```python
from build123d import *

# Parameters (mm, degrees)
SKETCH1_W           = 127
SKETCH1_H           = 38.1
BOSS_EXTRUDE1_DEPTH = 6.35
CUT_EXTRUDE1_DEPTH  = 6.35
FILLET1_R           = 30.48
CHAMFER1_SIZE       = 10.16
CHAMFER1_SIZE2      = 3.69793758


with BuildPart() as part:
    # Sketch1 → Boss-Extrude1 (new body)
    with BuildSketch(Plane.XY):
        with Locations((63.5, 19.05)):
            Rectangle(SKETCH1_W, SKETCH1_H)
    extrude(amount=BOSS_EXTRUDE1_DEPTH)

    # Sketch2 → Cut-Extrude1 (cut)
    with BuildSketch(Plane.XY.offset(6.35)):
        Polygon((12.7, 0), (30.660512242, 17.960512242), (96.339487758, 17.960512242), (114.3, 0), align=None)
    extrude(amount=-CUT_EXTRUDE1_DEPTH, mode=Mode.SUBTRACT)

    # Fillet1
    fillet1_edges = [part.edges().sort_by_distance(p)[0] for p in [
        (114.3, 0, 3.175),
        (12.7, 0, 3.175),
        (30.660512242, 17.960512242, 3.175),
        (96.339487758, 17.960512242, 3.175),
    ]]
    fillet(fillet1_edges, radius=FILLET1_R)

    # Chamfer1
    chamfer1_edges = [part.edges().sort_by_distance(p)[0] for p in [
        (63.5, 38.1, 0),
    ]]
    chamfer1_side = [part.faces().sort_by_distance(p)[0] for p in [
        (63.5, 24.04441534, 0),
    ]]
    chamfer(chamfer1_edges, length=CHAMFER1_SIZE, length2=CHAMFER1_SIZE2, reference=chamfer1_side[0])


solid = part.part
```
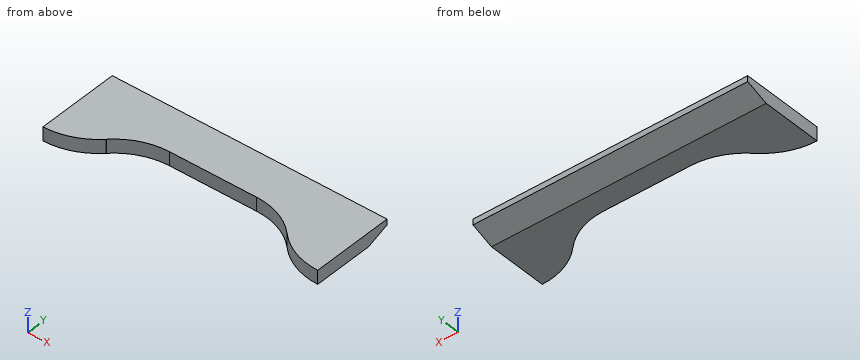
Geometry: final body of the model. Coordinates: model frame, mm. Coordinates: 2 decimals unless noted, no trailing zeros. Loops run counter-clockwise (first coordinate to the right, second up) from the corner with the lowest first, then second, coordinate; pieces in that order, holes last. Notation, with made-up numbers: M 71.25,22.5 L 94.25,22.5 A23 ccw 94.25,34.5 Z; hole C -40,41.25 d1. An arc over 180 degrees is marked long. Put each result on its own line as item: value.
(1) Cut plane B-B on y = 14. Return the cut outline in (x, z), then the cut area to 3 significant figures.
Answer sheet:
outline: M 0,0 L 28.26,0 L 28.26,6.35 L 0,6.35 Z; M 98.74,0 L 127,0 L 127,6.35 L 98.74,6.35 Z
area: 359 mm^2
(2) Cut plane C-C on x = 71. Return the cut outline in (y, z).
Answer sheet:
outline: M 17.96,0 L 27.94,0 L 38.1,3.7 L 38.1,6.35 L 17.96,6.35 Z
(3) Cut plane A-A on z = 5.25. Return the cut outline in (x, y).
Answer sheet:
outline: M 0,0 L 0.07,0 A30.48 ccw 21.63,8.93 L 21.73,9.03 A30.48 cw 43.29,17.96 L 83.71,17.96 A30.48 cw 105.27,9.03 L 105.37,8.93 A30.48 ccw 126.93,0 L 127,0 L 127,38.1 L 0,38.1 Z
(4) Material intervals for probe 1 along Y at (x, z) = (47, 5.25); probe 2 along X at (y, z) = (10, 3.5); probe 3 along X at (y, z) = (11.5, 6), sorted ascending.
Answer sheet:
probe 1: y = 17.96 to 38.1
probe 2: x = 0 to 22.75, 104.25 to 127
probe 3: x = 0 to 24.52, 102.48 to 127
(5) Cut plane D-D on y = 7.5. Return the cut outline in (x, z).
Answer sheet:
outline: M 0,0 L 20.1,0 L 20.1,6.35 L 0,6.35 Z; M 106.9,0 L 127,0 L 127,6.35 L 106.9,6.35 Z
(6) First-contact query: pin 1 (3 mm diameter, centred on x = 61.5, z = 2, fed in from -Y); pin 2 (10 mm diameter, centred on x = 50, y = 33, fed in from -Z). Flat tips, straight axial feed; report the tip coordinate or a pass-through.
Answer sheet:
pin 1: stops at y = 17.96
pin 2: stops at z = 0.02
